```python
from build123d import *

# Parameters (mm, degrees)
F1_DEPTH = 45.974
F2_SIZE  = 5.08
F3_R     = 5.08


with BuildPart() as f1:
    # F0 (on Front) → F1 (new body)
    with BuildSketch(Plane.XZ):
        with BuildLine():
            Line((0, 17.415097), (0, 0))
            Line((0, 0), (36.331072, 0))
            Line((36.331072, 0), (36.331072, 20.504786))
            ThreePointArc((36.331072, 20.504786), (46.944643, 46.128212), (21.321217, 35.514642))
            Line((21.321217, 35.514642), (18.099545, 35.514642))
            ThreePointArc((18.099545, 35.514642), (-12.798311, 48.312952), (0, 17.415097))
        make_face()
    extrude(amount=F1_DEPTH)

    # F2
    f2_edges = [f1.edges().sort_by_distance(p)[0] for p in [
        (0, -22.987, 0),
    ]]
    chamfer(f2_edges, length=F2_SIZE)

    # F3
    f3_edges = [f1.edges().sort_by_distance(p)[0] for p in [
        (36.331072, -22.987, 0),
    ]]
    fillet(f3_edges, radius=F3_R)


solid = f1.part
```
Could you check a few things on this model? Use its own coordinates, in mm. A direction names the side the tool comes from. Coordinates: 2 decimals unless noted, no trailing zeros. Order: outer loops, then holes, each group sorted by start corner. A loop starts at its lowest first (then second) coordinate and runs counter-clockwise, first axis right, second up. Notation, with made-up numbers: M 62,-22.5 L 108,-22.5 A20 cw 108,-14.5 Z; hole C 16.25,17 d4. An arc over 180 degrees is marked long. Use a Markdown table: item, result. Add a question column.
Q1. I want a section at A-A on y = -34. List the corners of the cut face in (x, z) for me, then the cut area to 3 significant figures.
Q2. I'm going to push flat-ended pins straight in: pin 1 (17 mm diameter, centred on y = -28.5, z = 10.5, fed in from +X); pin 2 (10 mm diameter, centred on y = -21.5, z = 21.5, fed in from -X); pin 3 (4 mm diameter, centred on y = -34.5, z = 45, fed in from -X). Where does each tip first touch, or does it pass through?
Q3. I want a section at C-C on z = 21.5. List the corners of the cut face in (x, y) for me, then the cut area to 3 significant figures.
Q4. We'd pull the mould along X, two halves only. Please class faces 1 (the flat face through (16, 0, 27)), 2 (the cylindrical face through (-12.4, -22.7, 48.7)), 3 (the cylindrical face through (34.803, -23.309, 1.449)): pulls with the +X half, pulls with the -X half, needs draft (parallel to the pull), parting line crosses it, or undercut.
Q5. Which directions (+Z, -Z, +X, -X, +Y, -Y) give clear straight access to the entire face, cutting with the end or side of a thin tool? Please do faces 4 (the flat face through (18, -23, 0)), 5 (the flat face through (0, -23, 11)), 6 (the flat face through (36.331, -23, 13)), 7 (the flat face through (20, -23, 35.515)), 8 (the flat face through (16, -45.974, 27)).
Q6. If I drill on L1, parallel to X at y = -29.5, z = 36; L2, parallel to X at y = -37.5, z = 6; L3, parallel to X at y = -4.5, z = 43.5, over which ranges is the centre line in solid material (lowest first)?
Q7. I want a section at B-B on x = 25.5. List the corners of the cut face in (y, z) for me, then the cut area to 3 significant figures.
Checked values:
| question | item | result |
|---|---|---|
| 1 | outline | M 0,5.08 L 5.08,0 L 31.25,0 A5.08 ccw 36.33,5.08 L 36.33,20.5 A15.01 ccw long 21.32,35.51 L 18.1,35.51 A18.1 ccw long 0,17.42 Z |
| 1 | area | 2,570 mm² |
| 2 | pin 1 | x = 36.33 |
| 2 | pin 2 | x = -15.69 |
| 2 | pin 3 | x = -16.48 |
| 3 | outline | M -11.45,-45.97 L 41.71,-45.97 L 41.71,0 L -11.45,0 Z |
| 3 | area | 2,440 mm² |
| 4 | face 1 | needs draft |
| 4 | face 2 | undercut |
| 4 | face 3 | pulls with the +X half |
| 5 | face 4 | -Z, +X, -X, +Y, -Y |
| 5 | face 5 | -Z, -X, +Y, -Y |
| 5 | face 6 | -Z, +X, +Y, -Y |
| 5 | face 7 | +Z, +Y, -Y |
| 5 | face 8 | +Z, -Z, +X, -X, -Y |
| 6 | L1 | -18.09 to 18.09, 21.33 to 51.33 |
| 6 | L2 | 0 to 36.33 |
| 6 | L3 | -16.24 to 16.24, 23.62 to 49.04 |
| 7 | outline | M -45.97,0 L 0,0 L 0,45.91 L -45.97,45.91 Z |
| 7 | area | 2,110 mm² |
